Part model, mm, in its own coordinate system. A direction names the side the tool comes from. Give positions to 0.01 mm unless a question says otherwise; leave off trailing zeros. Order: outer loops, then holes, each group sorted by start corner. A loop starts at its lowest first (then second) coordinate and runs counter-clockwise, first axis right, second up.
from build123d import *

# Parameters (mm, degrees)
F0_R        = 13.5
F0_R_2      = 9.3155
F1_DEPTH    = 11
F1_FACE_R   = 13.5
F1_FACE_R_2 = 9.3155
F4_R        = 13.5
F4_R_2      = 9.3155
F5_DEPTH    = 11


with BuildPart() as f1:
    # F0 (on Front) → F1 (new body)
    with BuildSketch(Plane.XZ):
        Circle(F0_R)
        Circle(F0_R_2, mode=Mode.SUBTRACT)
    extrude(amount=F1_DEPTH)

    # F3: sweep along a path in F2
    with BuildLine(Plane.YZ) as f3_path:
        ThreePointArc((0, 0), (11.313708, -4.686292), (16, -16))
    # F1_face (on face) → F3 (sweep)
    with BuildSketch(Plane(origin=(0, 0, 0), x_dir=(1, 0, 0), z_dir=(0, 1, 0))):
        Circle(F1_FACE_R)
        Circle(F1_FACE_R_2, mode=Mode.SUBTRACT)
    sweep(path=f3_path.line)

    # F4 (on face) → F5 (join)
    with BuildSketch(Plane(origin=(0, 0, -16), x_dir=(1, 0, 0), z_dir=(0, 0, -1))):
        with Locations((0, -16)):
            Circle(F4_R)
        with Locations((0, -16)):
            Circle(F4_R_2, mode=Mode.SUBTRACT)
    extrude(amount=F5_DEPTH)


solid = f1.part
Item 1: Band-saw the part on C-C on x = -6. List the corners of the cut face in (y, z), plus the area to 3 significant figures.
Item 2: Which spindle directions (+Z, -Z, +X, -X, +Y, -Y) get a long thin tool onto all of the face, cutting with end or side? Do faces 1 (the face through (9, -11, 3)), 2 (the face through (5.008, 8.145, -21.423)). Say none if no direction does.
Item 3: Band-saw the part on B-B on z = -18. List the corners of the cut face in (x, y), plus the area to 3 significant figures.
Item 4: Pull direction Z, two halves, no side cores. Call faces 3 (the face through (9, 13, -27)), 4 (the face through (-1.757, 2.615, -21.423)), 5 (the face through (8.885, -5.423, 2.798)), 6 (the face through (-2.93, -5.42, -13.18)): released by +Z, released by -Z, zero draft, split by the parting line, or undercut.
Item 5: Band-saw the part on D-D on x = 11.5. List the corners of the cut face in (y, z).
Item 6: Band-saw the part on A-A on x = 0. List the corners of the cut face in (y, z), plus the area to 3 significant figures.
Item 7: Drill centre lines: probe 1 along Y at (x, z) = (0, -22); probe 2 along X at (y, z) = (16, -21.75). Where is each one in solid material? Low to high.
Item 8: Drop flat-ended pins along their axis: P1, Ø1, axis at y = 18.5, z = -12.5, coming from the +X side; P2, Ø3, axis at x = 4.5, z = -4.5, coming from the -Y side (3 decimals); P3, Ø4, axis at y = 19, z = -4, coming from the -X side; P4, Ø4, axis at x = -4.5, z = 7.5, coming from the -Y side. Give the stop position or say it passes through.
Working result:
1. outline: (-11, -12.09) - (0, -12.09) arc R3.91 cw to (3.91, -16) - (3.91, -27) - (8.87, -27) - (8.87, -16) arc R8.87 ccw to (0, -7.13) - (-11, -7.13) - close; (-11, 7.13) - (0, 7.13) arc R23.13 cw to (23.13, -16) - (23.13, -27) - (28.09, -27) - (28.09, -16) arc R28.09 ccw to (0, 12.09) - (-11, 12.09) - close
1. area: 468 mm2
2. face 1: +Z, -Z, +X, -X, -Y
2. face 2: -Z
3. outline: circle Ø27 at (0, 16); hole circle Ø18.63 at (0, 16)
3. area: 300 mm2
4. face 3: released by -Z
4. face 4: zero draft
4. face 5: undercut
4. face 6: split by the parting line
5. outline: (-11, -7.07) - (0, -7.07) arc R8.93 cw to (8.93, -16) - (8.93, -27) - (23.07, -27) - (23.07, -16) arc R23.07 ccw to (0, 7.07) - (-11, 7.07) - close
6. outline: (-11, -13.5) - (0, -13.5) arc R2.5 cw to (2.5, -16) - (2.5, -27) - (6.68, -27) - (6.68, -16) arc R6.68 ccw to (0, -9.32) - (-11, -9.32) - close; (-11, 9.32) - (0, 9.32) arc R25.32 cw to (25.32, -16) - (25.32, -27) - (29.5, -27) - (29.5, -16) arc R29.5 ccw to (0, 13.5) - (-11, 13.5) - close
6. area: 394 mm2
7. probe 1: y = 2.5 to 6.68, 25.32 to 29.5
7. probe 2: x = -13.5 to -9.32, 9.32 to 13.5
8. P1: stops at x = 13.3
8. P2: stops at y = 19.805
8. P3: stops at x = -12.74
8. P4: stops at y = -11
